from build123d import *

# Parameters (mm, degrees)
BOSS_EXTRUDE4_DEPTH     = 50
CUT_EXTRUDE_THIN1_DEPTH = 50
BOSS_EXTRUDE6_DEPTH     = 7
BOSS_EXTRUDE8_START     = -7
BOSS_EXTRUDE8_DEPTH     = 7
BOSS_EXTRUDE9_START     = 7
BOSS_EXTRUDE9_DEPTH     = 7
SKETCH10_R              = 2
CUT_EXTRUDE1_DEPTH      = 59.576872569


with BuildPart() as part:
    # Sketch1 → Boss-Extrude4 (new body)
    with BuildSketch(Plane(origin=(0, 0, 0), x_dir=(0, 0, -1), z_dir=(1, 0, 0))):
        with BuildLine():
            Line((-25, 0), (-13, 0))
            ThreePointArc((-13, 0), (0, 13), (13, 0))
            Line((13, 0), (25, 0))
            ThreePointArc((25, 0), (0, 25), (-25, 0))
        make_face()
    extrude(amount=BOSS_EXTRUDE4_DEPTH)

    # Sketch4 → Cut-Extrude-Thin1 (cut)
    with BuildSketch(Plane.ZY.offset(-7)):
        with BuildLine():
            ThreePointArc((17.5, 0), (0, 17.5), (-17.5, 0))
            Line((-17.5, 0), (-27.5, 0))
            ThreePointArc((-27.5, 0), (0, 27.5), (27.5, 0))
            Line((27.5, 0), (17.5, 0))
        make_face()
    extrude(amount=-CUT_EXTRUDE_THIN1_DEPTH, mode=Mode.SUBTRACT)

    # Sketch5 → Boss-Extrude6 (add)
    with BuildSketch(Plane(origin=(7, 0, 0), x_dir=(0, 0, -1), z_dir=(1, 0, 0))):
        with BuildLine():
            Line((-19, 0), (-17.5, 0))
            ThreePointArc((-17.5, 0), (0, 17.5), (17.5, 0))
            Line((17.5, 0), (19, 0))
            ThreePointArc((19, 0), (0, 19), (-19, 0))
        make_face()
    extrude(amount=BOSS_EXTRUDE6_DEPTH)

    # Sketch8 → Boss-Extrude8 (add)
    with BuildSketch(Plane(origin=(50, 0, 0), x_dir=(0, 0, -1), z_dir=(1, 0, 0)).offset(BOSS_EXTRUDE8_START)):
        with BuildLine():
            Line((-25, 0), (-17.5, 0))
            ThreePointArc((-17.5, 0), (0, 17.5), (17.5, 0))
            Line((17.5, 0), (25, 0))
            ThreePointArc((25, 0), (0, 25), (-25, 0))
        make_face()
    extrude(amount=BOSS_EXTRUDE8_DEPTH)

    # Sketch9 → Boss-Extrude9 (add)
    with BuildSketch(Plane.ZY.offset(-43).offset(BOSS_EXTRUDE9_START)):
        with BuildLine():
            Line((-19, 0), (-17.5, 0))
            ThreePointArc((-17.5, 0), (0, 17.5), (17.5, 0))
            Line((17.5, 0), (19, 0))
            ThreePointArc((19, 0), (0, 19), (-19, 0))
        make_face()
    extrude(amount=-BOSS_EXTRUDE9_DEPTH)

    # Sketch10 → Cut-Extrude1 (cut, through all)
    with BuildSketch(Plane(origin=(0, 17.5, 0), x_dir=(1, 0, 0), z_dir=(0, 1, 0))):
        with Locations(Location((25, 0, 0), (0, 0, 270))):
            Circle(SKETCH10_R)
    extrude(amount=-CUT_EXTRUDE1_DEPTH, mode=Mode.SUBTRACT)


solid = part.part
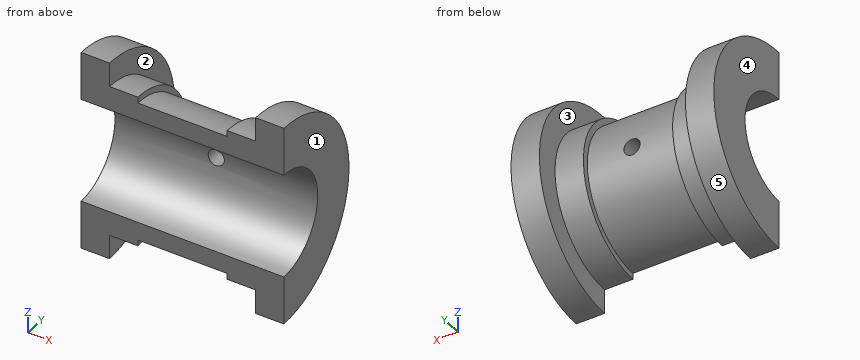
Work out the finished part from the listing and answer in its coordinate system (mm). Face numbers are marked on the shaded views. A direction names the side the tool comes from. Coordinates: 2 decimals unless noted, no trailing zeros. Write each loop counter-clockwise with the first axis right and the second up, starting at its lowest first coordinate (ties: lowest second). Pieces come first, ordered by that corner, then holes.
1. The part is cut by section C-C, the plane x = 25. Write down the section's boundary in (y, z).
Results list:
outline: (0, -17.5) arc R17.5 ccw to (17.39, -2) - (12.85, -2) arc R13 cw to (0, -13) - close; (0, 13) arc R13 cw to (12.85, 2) - (17.39, 2) arc R17.5 ccw to (0, 17.5) - close
2. The part is cut by section D-D, the plane z = -6. Write down the section's boundary in (x, y).
Results list:
outline: (0, 11.53) - (50, 11.53) - (50, 24.27) - (43, 24.27) - (43, 18.03) - (36, 18.03) - (36, 16.44) - (14, 16.44) - (14, 18.03) - (7, 18.03) - (7, 24.27) - (0, 24.27) - close
3. For the marked faces 1 and 2, determine the directions among +Z, -Z, +X, -X, +Y, -Y from which every point of the face is accessible in a straight line to the end or side of a thin tool.
Results list:
face 1: +Z, -Z, +X, +Y, -Y
face 2: +Y
4. Flat-ended cylindrical pins translate along their axes: pin 1 (6 mm diameter, centred on x = 31, y = 13.5, fed in from +Z); pin 2 (10 mm diameter, centred on x = 35, z = -6, fed in from +Y); pin 3 (4.5 mm diameter, centred on x = 25, z = 0, fed in from +Y). Find the tip coordinate at first contact, or state that the pin passes through.
Results list:
pin 1: stops at z = 14
pin 2: stops at y = 18.97
pin 3: stops at y = 17.5
5. Consider line 1 along X through (y, z) = (18.5, -6); line 2 along X through (y, z) = (15.05, 0); line 3 along Z through (x, y) = (25, 14.6). Determine where each line is inside the solid, lowest interval first.
Results list:
line 1: x = 0 to 7, 43 to 50
line 2: x = 0 to 23, 27 to 50
line 3: z = -9.65 to -2, 2 to 9.65
6. For a pull along X with two mould halves and no side action, classify the marked faces 3, 4 and 5 as +X half, -X half, draft (parallel to the pull), parting line (faces both ways), or undercut.
Results list:
face 3: undercut
face 4: -X half
face 5: draft
7. The part is cut by section B-B, the plane y = 20.75. Write down the section's boundary in (x, z).
Results list:
outline: (0, -13.94) - (7, -13.94) - (7, 13.94) - (0, 13.94) - close; (43, -13.94) - (50, -13.94) - (50, 13.94) - (43, 13.94) - close
8. The part is cut by section A-A, the plane z = 0. Write down the section's boundary in (x, y).
Results list:
outline: (0, 13) - (23, 13) - (23, 17.5) - (14, 17.5) - (14, 19) - (7, 19) - (7, 25) - (0, 25) - close; (27, 13) - (50, 13) - (50, 25) - (43, 25) - (43, 19) - (36, 19) - (36, 17.5) - (27, 17.5) - close
